```python
from build123d import *

# Parameters (mm, degrees)
F1_DEPTH = 50
F2_DEPTH = 100
F3_R     = 12.5
F4_DEPTH = 100


with BuildPart() as f1:
    # F0 (on Top) → F1 (new body)
    with BuildSketch(Plane.XY):
        with BuildLine():
            ThreePointArc((-27.848724, 0), (-10.399488, 12.464069), (-3.718301, 32.840295))
            ThreePointArc((-3.718301, 32.840295), (-58.332346, 60.698612), (-48.823562, 0.131601))
            ThreePointArc((-48.823562, 0.131601), (-38.346414, -1.571236), (-27.848724, 0))
        make_face()
    extrude(amount=F1_DEPTH)

    # F0 (on Top) → F2 (join)
    with BuildSketch(Plane.XY):
        with BuildLine():
            ThreePointArc((-27.848724, 0), (-38.346414, -1.571236), (-48.823562, 0.131601))
            Line((-48.823562, 0.131601), (-48.823562, -61.224833))
            Line((-48.823562, -61.224833), (-27.848724, -61.224833))
            Line((-27.848724, -61.224833), (-27.848724, 0))
        make_face()
    extrude(amount=F2_DEPTH)

    # F3 (on face) → F4 (cut)
    with BuildSketch(Plane.XY.offset(50)):
        with Locations((-38.130508, 32.840295)):
            Circle(F3_R)
    extrude(amount=-F4_DEPTH, mode=Mode.SUBTRACT)


solid = f1.part
```
Geometry: final body of the model. Coordinates: model frame, mm. A direction names the side the tool comes from. Round coordinates to 2 decimals unless told otherwise and drop trailing zeros. Write each loop counter-clockwise with the first axis right and the second up, starting at its lowest first coordinate (ties: lowest second). Pieces come first, ordered by that corner, then holes.
Item 1: Material intervals for L1, parallel to X at y = -31.5, z = 29; L2, parallel to Z at x = -64, y = 22.5; L3, parallel to Y at x = -35, z = 58, sorted ascending.
Item 2: Section query A-A (x = -36.5). Return loops of the section in (y, z), plus the area to 3 significant figures.
Item 3: Section query B-B (y = 30.5). Return loops of the section in (x, z).
Item 4: Section query C-C (z = 14.5). Return loops of the section in (x, y), plus the area to 3 significant figures.
Item 5: Section query D-D (y = -10). Return loops of the section in (x, z).
Item 6: Pin query (flat end, axial travel): P1, Ø20.5, axis at x = -34.5, y = 23.5, coming from the +Z side; P2, Ø2, axis at x = -54.5, z = 21, coming from the -Y side; P3, Ø6, axis at y = 25.5, z = 34, coming from the -X side. Return the tip coordinate at first contact, or that it passes through.
Item 7: Mould query, pull axis X, two halves, no side actions, for faces 1 (the face through (-38, -61.225, 49)), 2 (the face through (-48.824, -30, 49)), 3 (the face through (-26.584, 28.053, 25.35)). Classes: +X half, -X half, draft (parallel to the pull), parting line (faces both ways), or undercut.
Item 8: Set-up query: faces 4 (the face through (-27.849, -31, 49)), 5 (the face through (-38.2, -1.57, 74.65)), 6 (the face through (-39, 18, 0)). Return all of +Z, -Z, +X, -X, +Y, -Y with unobstructed straight access to the full face (end or side cutting, diameter ignored); none if empty.
Completed:
1. L1: x = -48.82 to -27.85
1. L2: z = 0 to 50
1. L3: y = -61.22 to -1.43
2. outline: (-61.22, 0) - (20.45, 0) - (20.45, 50) - (-1.53, 50) - (-1.53, 100) - (-61.22, 100) - close; (45.23, 0) - (67.21, 0) - (67.21, 50) - (45.23, 50) - close
2. area: 8,170 mm2
3. outline: (-72.46, 0) - (-50.41, 0) - (-50.41, 50) - (-72.46, 50) - close; (-25.85, 0) - (-3.8, 0) - (-3.8, 50) - (-25.85, 50) - close
4. outline: (-48.82, -61.22) - (-27.85, -61.22) - (-27.85, 0) arc R34.41 ccw to (-3.72, 32.84) arc R34.41 ccw (long way) to (-48.82, 0.13) - close; hole circle Ø25 at (-38.13, 32.84)
4. area: 4,490 mm2
5. outline: (-48.82, 0) - (-27.85, 0) - (-27.85, 100) - (-48.82, 100) - close
6. P1: stops at z = 50
6. P2: stops at y = 2.05
6. P3: stops at x = -72.27
7. face 1: draft
7. face 2: -X half
7. face 3: undercut
8. face 4: +Z, -Z, +X, -Y
8. face 5: +Z, +Y
8. face 6: -Z, +X, -X, +Y, -Y
